```python
from build123d import *

# Parameters (mm, degrees)
F1_DEPTH = 400
F2_W     = 350
F2_H     = 300
F3_DEPTH = 400.001


with BuildPart() as f1:
    # F0 (on Top) → F1 (new body)
    with BuildSketch(Plane.XY):
        Polygon((-200, -200), (200, -200), (200, 200), (150, 200), (150, -150), (-150, -150), (-150, 200), (-200, 200), align=None)
    extrude(amount=F1_DEPTH)

    # F2 (on face) → F3 (cut, through all)
    with BuildSketch(Plane(origin=(-200, 0, 0), x_dir=(0, -1, 0), z_dir=(-1, 0, 0))):
        with Locations((-25, 200)):
            Rectangle(F2_W, F2_H)
    extrude(amount=-F3_DEPTH, mode=Mode.SUBTRACT)


solid = f1.part
```
Source: CAD feature listing. Evaluate the final solid. Frame: model axes, mm. A direction names the side the tool comes from. Round coordinates to 2 decimals unless told otherwise and drop trailing zeros. Loops run counter-clockwise (first coordinate to the right, second up) from the corner with the lowest first, then second, coordinate; pieces in that order, holes last. Notation, with made-up numbers: M 44,35 L 68,35 A20 ccw 68,44 Z; hole C 52,77.25 d2. An arc over 180 degrees is marked long. Use a Markdown table: item, result. Add a question column.
1. Reachability of faces 4 (the flat face through (175, 27, 350)), 5 (the flat face through (150, 27, 375)), 6 (the flat face through (-1, -162, 400)) from +Z, -Z, +X, -X, +Y, -Y: full face, straight path, thin tool, end or side. Return the list, or none.
2. Mould query, pull axis X, two halves, no side actions, for faces 1 (the flat face through (-3, -150, 197)), 2 (the flat face through (-175, 200, 375)), 3 (the flat face through (-200, -162, 214)). Classes: pulls with the +X half, pulls with the -X half, needs draft (parallel to the pull), parting line crosses it, or undercut.
3. Line query: line 1 (Z direction, x = -181.5, y = 132); line 2 (X direction, y = 19, z = 45); line 3 (Y direction, x = 80.5, z = 150). Output: solid intervals per line, ascending.
4. Section query C-C on x = -124.5. Return the cut outline in (y, z).
5. Section query A-A on y = -29. Return the cut outline in (x, z).
6. Section query B-B on z = 151.5. Return the cut outline in (x, y), then the cut area to 3 significant figures.
7. Contact query for flat-ended pins moving along their axis: P1, Ø3, axis at x = 23.5, z = 247, coming from the +Y side; P2, Ø25, axis at x = -169, y = 74, coming from the -Z side. Output: stop coordinate, or through.
Reported:
| question | item | result |
|---|---|---|
| 1 | face 4 | +X, -X, +Y |
| 1 | face 5 | +Z, -Z, +Y |
| 1 | face 6 | +Z, +X, -X, +Y, -Y |
| 2 | face 1 | undercut |
| 2 | face 2 | needs draft |
| 2 | face 3 | pulls with the -X half |
| 3 | line 1 | z = 0 to 50, 350 to 400 |
| 3 | line 2 | x = -200 to -150, 150 to 200 |
| 3 | line 3 | y = -200 to -150 |
| 4 | outline | M -200,0 L -150,0 L -150,400 L -200,400 Z |
| 5 | outline | M -200,0 L -150,0 L -150,50 L -200,50 Z; M -200,350 L -150,350 L -150,400 L -200,400 Z; M 150,0 L 200,0 L 200,50 L 150,50 Z; M 150,350 L 200,350 L 200,400 L 150,400 Z |
| 6 | outline | M -200,-200 L 200,-200 L 200,-150 L -200,-150 Z |
| 6 | area | 20,000 mm² |
| 7 | P1 | stops at y = -150 |
| 7 | P2 | stops at z = 0 |
